Design review of the part built by this model. Coordinates are the model's own, in mm. A direction names the side the tool comes from. Give positions to 0.01 mm unless a question says otherwise; leave off trailing zeros. Write each loop counter-clockwise with the first axis right and the second up, starting at its lowest first coordinate (ties: lowest second). Pieces come first, ordered by that corner, then holes. Notation, with made-up numbers: M -24,78.25 L 9,78.25 A34 cw 9,110.25 Z; hole C 8.5,-9.75 d8. An arc over 180 degrees is marked long. Write each question's results on one line, items separated by ' | '. Start each with the question number.
from build123d import *

# Parameters (mm, degrees)
CYLINDER016030_R            = 3.15
CYLINDER016030_DEPTH        = 10
CYLINDER_R                  = 4.1
CYLINDER_DEPTH              = 36
CYLINDER003_R               = 0.85
CYLINDER003_DEPTH           = 10
CYLINDER004_R               = 2.5
CYLINDER004_DEPTH           = 3
CYLINDER002_R               = 3.15
CYLINDER002_DEPTH           = 33
CYLINDER001_R               = 6.5
CYLINDER001_DEPTH           = 33
BOX013_W                    = 3.5
BOX013_H                    = 10
BOX013_DEPTH                = 43
BOX001_W                    = 10
BOX001_H                    = 28
BOX001_DEPTH                = 40
CHAMFER_SIZE                = 3
CHAMFER016009_SIZE          = 5
CHAMFER016013_SIZE          = 0.4
BOX003_W                    = 6
BOX003_H                    = 7.8
BOX003_DEPTH                = 20
BOX002_W                    = 2
BOX002_H                    = 7.8
BOX002_DEPTH                = 40
CHAMFER005_SIZE             = 1
BOX014_W                    = 3.5
BOX014_H                    = 10
BOX014_DEPTH                = 43
BOX_W                       = 24
BOX_H                       = 28
BOX_DEPTH                   = 20
CHAMFER016010_SIZE          = 5
CHAMFER016014_SIZE          = 1
CHAMFER016015_SIZE          = 0.4
CHAMFER016016_SIZE          = 0.4
CHAMFER016016008004017_SIZE = 0.4


with BuildPart() as cylinder044:
    # Cylinder016030 → Cylinder016030 (new body)
    with BuildSketch(Plane(origin=(20.5, 12, 10), x_dir=(0, 0, -1), z_dir=(1, 0, 0))):
        Circle(CYLINDER016030_R)
    extrude(amount=CYLINDER016030_DEPTH)


with BuildPart() as cylinder:
    # Cylinder → Cylinder (new body)
    with BuildSketch(Plane(origin=(14, 4.5, 10), x_dir=(1, 0, 0), z_dir=(0, 1, 0))):
        Circle(CYLINDER_R)
    extrude(amount=CYLINDER_DEPTH)


with BuildPart() as cylinder003:
    # Cylinder003 → Cylinder003 (new body)
    with BuildSketch(Plane(origin=(10, 20, 0), x_dir=(1, 0, 0), z_dir=(0, 0, 1))):
        Circle(CYLINDER003_R)
    extrude(amount=CYLINDER003_DEPTH)


with BuildPart() as fusion003:
    # Cylinder004 → Cylinder004 (new body)
    with BuildSketch(Plane(origin=(10, 20, 0), x_dir=(1, 0, 0), z_dir=(0, 0, 1))):
        Circle(CYLINDER004_R)
    extrude(amount=CYLINDER004_DEPTH)

    # Fusion003: union Cylinder003
    add(cylinder003.part)


with BuildPart() as fusion003_1:
    # Fusion003 placement: moved
    add(fusion003.part.moved(Location((4, 0, 0))))


with BuildPart() as cylinder002:
    # Cylinder002 → Cylinder002 (new body)
    with BuildSketch(Plane(origin=(-10, 15, 30), x_dir=(0, 0, -1), z_dir=(1, 0, 0))):
        Circle(CYLINDER002_R)
    extrude(amount=CYLINDER002_DEPTH)


with BuildPart() as fusion005:
    # Cylinder001 → Cylinder001 (new body)
    with BuildSketch(Plane(origin=(8, 15, 30), x_dir=(0, 0, -1), z_dir=(1, 0, 0))):
        Circle(CYLINDER001_R)
    extrude(amount=CYLINDER001_DEPTH)

    # Fusion005: union Cylinder002
    add(cylinder002.part)


with BuildPart() as cube013:
    # Box013 → Box013 (new body)
    with BuildSketch(Plane(origin=(0, 22.5, 0), x_dir=(1, 0, 0), z_dir=(0, 0, 1))):
        with Locations((1.75, 5)):
            Rectangle(BOX013_W, BOX013_H)
    extrude(amount=BOX013_DEPTH)


with BuildPart() as chamfer016013:
    # Box001 → Box001 (new body)
    with BuildSketch(Plane(origin=(0, 2, 0), x_dir=(1, 0, 0), z_dir=(0, 0, 1))):
        with Locations((5, 14)):
            Rectangle(BOX001_W, BOX001_H)
    extrude(amount=BOX001_DEPTH)

    # Chamfer
    chamfer_edges = [chamfer016013.edges().sort_by_distance(p)[0] for p in [
        (5, 2, 40),
    ]]
    chamfer(chamfer_edges, length=CHAMFER_SIZE)

    # Chamfer016009
    chamfer016009_edges = [chamfer016013.edges().sort_by_distance(p)[0] for p in [
        (5, 30, 40),
    ]]
    chamfer(chamfer016009_edges, length=CHAMFER016009_SIZE)

    # Cut010011002: cut Cube013
    add(cube013.part, mode=Mode.SUBTRACT)

    # Chamfer016013
    chamfer016013_edges = [chamfer016013.edges().sort_by_distance(p)[0] for p in [
        (0, 13.75, 40),
        (0, 12.25, 0),
        (0, 2, 18.5),
        (0, 3.5, 38.5),
        (10, 15, 40),
        (1.75, 22.5, 0),
        (3.5, 26.25, 0),
        (6.75, 30, 0),
        (10, 16, 0),
        (10, 2, 18.5),
        (10, 3.5, 38.5),
        (10, 27.5, 37.5),
        (10, 30, 17.5),
    ]]
    chamfer(chamfer016013_edges, length=CHAMFER016013_SIZE)


with BuildPart() as cube003:
    # Box003 → Box003 (new body)
    with BuildSketch(Plane(origin=(-5, 11.1, 0), x_dir=(1, 0, 0), z_dir=(0, 0, 1))):
        with Locations((3, 3.9)):
            Rectangle(BOX003_W, BOX003_H)
    extrude(amount=BOX003_DEPTH)


with BuildPart() as chamfer005:
    # Box002 → Box002 (new body)
    with BuildSketch(Plane(origin=(-1, 11.1, 0), x_dir=(1, 0, 0), z_dir=(0, 0, 1))):
        with Locations((1, 3.9)):
            Rectangle(BOX002_W, BOX002_H)
    extrude(amount=BOX002_DEPTH)

    # Fusion: union Cube003
    add(cube003.part)

    # Chamfer005
    chamfer005_edges = [chamfer005.edges().sort_by_distance(p)[0] for p in [
        (-5, 15, 0),
        (-1, 15, 40),
        (-5, 15, 20),
    ]]
    chamfer(chamfer005_edges, length=CHAMFER005_SIZE)


with BuildPart() as cube014:
    # Box014 → Box014 (new body)
    with BuildSketch(Plane(origin=(0, 22.5, 0), x_dir=(1, 0, 0), z_dir=(0, 0, 1))):
        with Locations((1.75, 5)):
            Rectangle(BOX014_W, BOX014_H)
    extrude(amount=BOX014_DEPTH)


with BuildPart() as rod_mount_front_w_magnet:
    # Box → Box (new body)
    with BuildSketch(Plane(origin=(0, 2, 0), x_dir=(1, 0, 0), z_dir=(0, 0, 1))):
        with Locations((12, 14)):
            Rectangle(BOX_W, BOX_H)
    extrude(amount=BOX_DEPTH)

    # Chamfer016010
    chamfer016010_edges = [rod_mount_front_w_magnet.edges().sort_by_distance(p)[0] for p in [
        (24, 2, 10),
    ]]
    chamfer(chamfer016010_edges, length=CHAMFER016010_SIZE)

    # Chamfer016014
    chamfer016014_edges = [rod_mount_front_w_magnet.edges().sort_by_distance(p)[0] for p in [
        (24, 30, 10),
    ]]
    chamfer(chamfer016014_edges, length=CHAMFER016014_SIZE)

    # Cut: cut Cube014
    add(cube014.part, mode=Mode.SUBTRACT)

    # Chamfer016015
    chamfer016015_edges = [rod_mount_front_w_magnet.edges().sort_by_distance(p)[0] for p in [
        (24, 18, 20),
        (24, 18, 0),
        (21.5, 4.5, 20),
        (9.5, 2, 20),
        (0, 12.25, 20),
        (1.75, 22.5, 20),
        (3.5, 26.25, 20),
        (13.25, 30, 20),
        (23.5, 29.5, 20),
        (23.5, 29.5, 0),
        (21.5, 4.5, 0),
        (9.5, 2, 0),
        (0, 12.25, 0),
        (1.75, 22.5, 0),
        (3.5, 26.25, 0),
        (13.25, 30, 0),
    ]]
    chamfer(chamfer016015_edges, length=CHAMFER016015_SIZE)

    # Fusion016: union Chamfer016013, Chamfer005
    add(chamfer016013.part)
    add(chamfer005.part)

    # Cut010011003: cut Fusion005
    add(fusion005.part, mode=Mode.SUBTRACT)

    # Cut010011004: cut Fusion003
    add(fusion003_1.part, mode=Mode.SUBTRACT)

    # Cut010011005: cut Cylinder
    add(cylinder.part, mode=Mode.SUBTRACT)

    # Chamfer016016
    chamfer016016_edges = [rod_mount_front_w_magnet.edges().sort_by_distance(p)[0] for p in [
        (9.9, 30, 10),
    ]]
    chamfer(chamfer016016_edges, length=CHAMFER016016_SIZE)

    # Cut010011008009003016002: cut Cylinder044
    add(cylinder044.part, mode=Mode.SUBTRACT)

    # Chamfer016016008004017
    chamfer016016008004017_edges = [rod_mount_front_w_magnet.edges().sort_by_distance(p)[0] for p in [
        (24, 12, 13.15),
    ]]
    chamfer(chamfer016016008004017_edges, length=CHAMFER016016008004017_SIZE)


solid = rod_mount_front_w_magnet.part
Q1. Wall thickness on line 1 along Y through (x, z) = (14, 1.25); line 2 along X through (y, z) = (5.5, 10); line 3 along Y through (x, z) = (2, 30): over which ranges is each line inside the solid? List them lowest first. Write a range as from..to.
Q2. For pin 1 Ø1 at (y, z) = (24.5, 11) entering from -X; pin 2 Ø2.5 at (x, y) = (14.5, 19) entering from -Z; pin 3 Ø5 at (y, z) = (15, 30) entering from +X; pin 4 Ø8.5 at (y, z) = (13.5, 30.5) entering from -X, all flat-tipped, find the tip position at first contact; note any pin that passes through.
Q3. The part is to be moulded in two halves that separate along Z. For faces 1 (the cylindrical face through (8.986, 15.286, 36.494)), 2 (the flat face through (-5, 15, 10)), 3 (the cylindrical face through (22.03, 14.13, 12.32)), 4 (the flat face through (21.326, 4.604, 0.203)), say which applies: pulls with the +Z half, pulls with the -Z half, needs draft (parallel to the pull), parting line crosses it, or undercut.
Q4. We need section D-D on x = 4.75. Write out the cut boundary in (y, z).
Q5. For faces 5 (the flat face through (17, 16, 20)), 6 (the flat face through (-1, 13, 27)), 7 (the cylindrical face through (12.16, 21.69, 1.48)), 8 (the flat face through (0, 6, 20)), list the 3-axis set-ups (+Z, -Z, +X, -X, +Y, -Y) from which the entire face can be reached by the end or side of a thin tool; tool diameter is ignored.
Q6. We need section B-B on y = 24. Write out the cut boundary in (x, z).
Q7. We need section A-A on x = 14. Write out the cut boundary in (y, z).
Q8. We need section C-C on z = 30. Write out the cut boundary in (x, y), and give its area (3 significant figures).
Answer sheet:
1) line 1: 2..17.5, 22.5..30 | line 2: 0..9.9, 18.1..22.5 | line 3: 2..11.85, 18.15..22.5
2) pin 1: x = 3.5 | pin 2: z = 3 | pin 3: through | pin 4: x = -1
3) face 1: undercut | face 2: needs draft | face 3: undercut | face 4: pulls with the -Z half
4) outline: M 2,0 L 29.6,0 L 30,0.4 L 30,35 L 25,40 L 5,40 L 2,37 Z; hole C 15,30 d6.3
5) face 5: +Z, +X, +Y, -Y | face 6: +Z, -X, +Y, -Y | face 7: -Z | face 8: +Z, -Z, -X, -Y
6) outline: M 3.5,0.4 L 3.9,0 L 23.6,0 L 24,0.4 L 24,19.6 L 23.6,20 L 10,20 L 10,39.6 L 9.6,40 L 3.5,40 Z; hole C 14,10 d8.2
7) outline: M 2,0.4 L 2.4,0 L 17.5,0 L 17.5,3 L 19.15,3 L 19.15,5.9 L 4.5,5.9 L 4.5,14.1 L 29.6,14.1 L 30,14.5 L 30,19.6 L 29.6,20 L 2.4,20 L 2,19.6 Z; M 20.85,3 L 22.5,3 L 22.5,0 L 29.6,0 L 30,0.4 L 30,5.5 L 29.6,5.9 L 20.85,5.9 Z
8) outline: M -1,11.1 L 0,11.1 L 0,2.4 L 0.4,2 L 9.6,2 L 10,2.4 L 10,8.5 L 8,8.5 L 8,11.85 L -1,11.85 Z; M -1,18.15 L 8,18.15 L 8,21.5 L 10,21.5 L 10,29.6 L 9.6,30 L 3.5,30 L 3.5,22.5 L 0,22.5 L 0,18.9 L -1,18.9 Z | area: 179 mm^2
